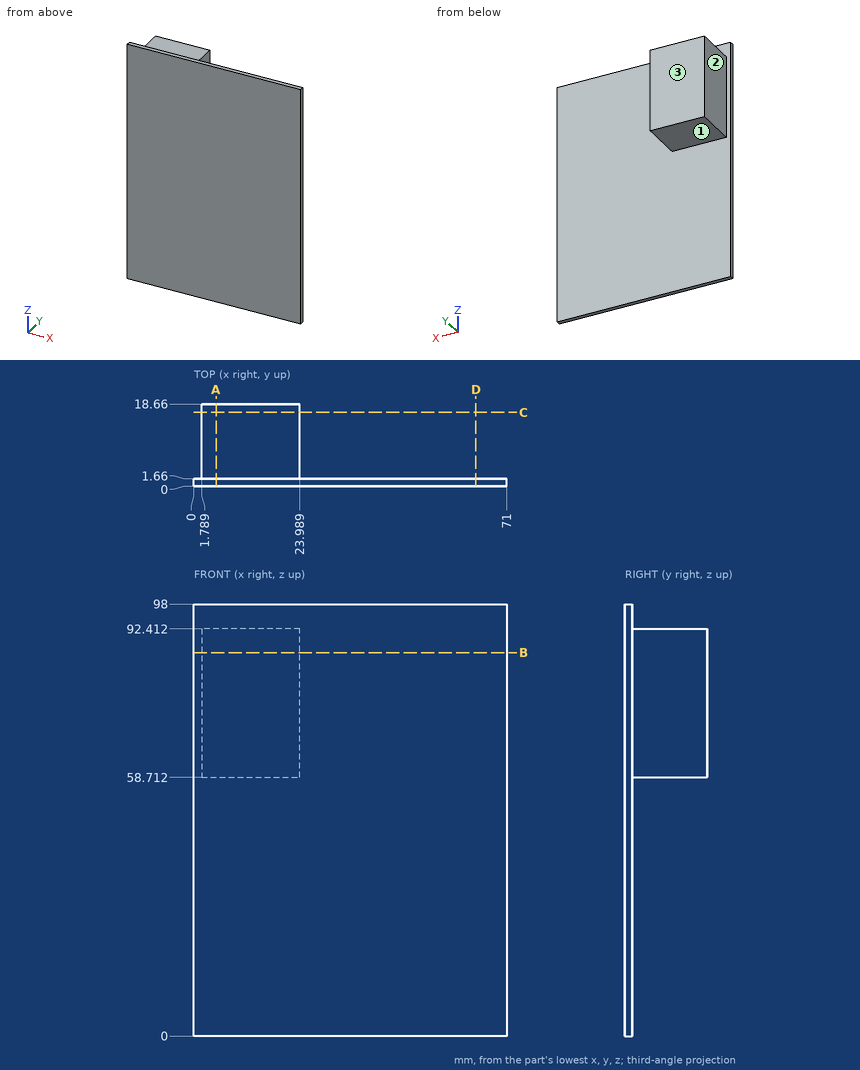
Verification items for this drawing (mm, ordinates from the low corner). A direction names the side the tool comes from. Give positions to 0.01 mm unless a question says otherwise; leave off trailing zeros. Order: outer loops, then holes, each group sorted by start corner. A loop starts at its lowest first (then second) coordinate and runs counter-clockwise, first axis right, second up. Notation, with made-up numbers: M 5,-22 L 27,-22 A28 ccw 27,-4 Z; hole C -18.5,-39.5 d2. An arc over 180 degrees is marked long. Use a Markdown table: item, result.
Item 1: Section check B-B (z = 87). Record the cut outline in (x, y), and give its area (3 significant figures).
Answers follow:
| item | result |
|---|---|
| outline | M 0,0 L 71,0 L 71,1.66 L 23.99,1.66 L 23.99,18.66 L 1.79,18.66 L 1.79,1.66 L 0,1.66 Z |
| area | 495 mm2 |
Item 2: Material ranges on line 1 along X through (y, z) = (15.5, 79); line 2 along Y through (x, z) = (40, 48); line 3 along Z through (x, y) = (16.5, 12), recorded low to high.
Answers follow:
| item | result |
|---|---|
| line 1 | x = 1.79 to 23.99 |
| line 2 | y = 0 to 1.66 |
| line 3 | z = 58.71 to 92.41 |
Item 3: Tool access check on the marked faces 1, 2 and 3. Record the directions out of +Z, -Z, +X, -X, +Y, -Y that give a thin tool (end or side, any length) a straight path to the whole face; none if there is none.
Answers follow:
| item | result |
|---|---|
| face 1 | -Z, +X, -X, +Y |
| face 2 | +Z, -Z, -X, +Y |
| face 3 | +Z, -Z, +X, -X, +Y |
Item 4: Section check A-A (x = 5). Record the cut outline in (y, z).
Answers follow:
| item | result |
|---|---|
| outline | M 0,0 L 1.66,0 L 1.66,58.71 L 18.66,58.71 L 18.66,92.41 L 1.66,92.41 L 1.66,98 L 0,98 Z |
Item 5: Section check D-D (x = 64). Record the cut outline in (y, z).
Answers follow:
| item | result |
|---|---|
| outline | M 0,0 L 1.66,0 L 1.66,98 L 0,98 Z |
Item 6: Section check C-C (y = 16.75). Record the cut outline in (x, z), and give its area (3 significant figures).
Answers follow:
| item | result |
|---|---|
| outline | M 1.79,58.71 L 23.99,58.71 L 23.99,92.41 L 1.79,92.41 Z |
| area | 748 mm2 |
Item 7: Depth check by flat-ended pin: P1, Ø8.5, axis at y = 11.5, z = 76, coming from the +X side; P2, Ø1, axis at x = 15, y = 8, coming from the +Z side; P3, Ø8.5, axis at y = 13.5, z = 69.5, coming from the -X side; P4, Ø6, axis at y = 7.5, z = 16, coming from the +X side. Enter the tip coordinate at first touch or a pass-through.
Answers follow:
| item | result |
|---|---|
| P1 | stops at x = 23.99 |
| P2 | stops at z = 92.41 |
| P3 | stops at x = 1.79 |
| P4 | passes through |
